Check sheet for the modelled part. Datum: model origin and axes. Units: mm. Face numbers are marked on the shaded views. A direction names the side the tool comes from. Give positions to 0.01 mm unless a question says otherwise; leave off trailing zeros. Loops run counter-clockwise (first coordinate to the right, second up) from the corner with the lowest first, then second, coordinate; pieces in that order, holes last. Notation, with made-up numbers: M 73.5,89.5 L 87.5,89.5 A27 cw 87.5,128.5 Z; hole C 74.25,-22.5 d11. An arc over 180 degrees is marked long. Write each question's results on one line, items separated by ' | '. Start each with the question number.
1. Sectioned sample at C-C on y = 54. Record the cut outline in (x, z), and give its area (3 significant figures).
2. Draft check along Z on the marked faces 3 and 4. Enter one of: pulls with the +Z half, pulls with the -Z half, needs draft (parallel to the pull), parting line crosses it, or undercut.
3. Tool access check on the marked faces 1 and 2. Record the directions out of +Z, -Z, +X, -X, +Y, -Y that give a thin tool (end or side, any length) a straight path to the whole face; none if there is none.
4. Sectioned sample at B-B on z = 20. Record the cut outline in (x, y), and give its area (3 significant figures).
5. Sectioned sample at D-D on x = -20. Record the cut outline in (y, z), and give its area (3 significant figures).
6. Sectioned sample at A-A on x = 0. Give the number of separate pieces and of enclosed holes in the cut face, and give its area (3 significant figures).
7. Material ranges on line 1 along X through (y, z) = (124.9, 0); line 2 along X through (y, z) = (39.5, 0); line 3 along Y through (x, z) = (22, 1), recorded low to high.
8. Go/stop test with flat-tipped pins: pin 1 (10 mm diameter, centred on x = 12, y = 100, fed in from -Z); pin 2 (15.5 mm diameter, centred on x = 0, z = 0, fed in from -Y); pin 3 (3 mm diameter, centred on x = -9.5, y = 84, fed in from +Z). Record where each tip stops, or that it passes through.
```python
from build123d import *

# Parameters (mm, degrees)
SKETCH2_R           = 37.5
BOSS_EXTRUDE1_DEPTH = 2
SKETCH4_R           = 15
BOSS_EXTRUDE2_DEPTH = 61
SKETCH5_R           = 25
BOSS_EXTRUDE3_DEPTH = 3
CUT_EXTRUDE1_REACH  = 139.628
SKETCH6_R           = 1.5
CUT_EXTRUDE2_REACH  = 139.628
SKETCH7_R           = 1.5
SHELL1_OUTLINE_R    = 13
SHELL1_DEPTH        = 125


# Read off the part's stored shape, not the designer's step: Shell1
with BuildPart() as part:
    # Sketch2 → Boss-Extrude1 (new body)
    with BuildSketch(Plane(origin=(0, 0, 0), x_dir=(1, 0, 0), z_dir=(0, 1, 0))):
        with Locations(Location((0, 0, 0), (0, 0, 270))):
            Circle(SKETCH2_R)
    extrude(amount=BOSS_EXTRUDE1_DEPTH)

    # Sketch4 → Boss-Extrude2 (add)
    with BuildSketch(Plane(origin=(0, 2, 0), x_dir=(1, 0, 0), z_dir=(0, 1, 0))):
        with Locations(Location((0, 0, 0), (0, 0, 90))):
            Circle(SKETCH4_R)
    boss_extrude2 = extrude(amount=BOSS_EXTRUDE2_DEPTH)

    # Mirror1: Boss-Extrude2 across plane
    add(boss_extrude2.mirror(Plane.ZX.offset(63)))

    # Sketch5 → Boss-Extrude3 (add)
    with BuildSketch(Plane(origin=(0, 124, 0), x_dir=(1, 0, 0), z_dir=(0, 1, 0))):
        with Locations(Location((0, 0, 0), (0, 0, 270))):
            Circle(SKETCH5_R)
    extrude(amount=BOSS_EXTRUDE3_DEPTH)

    # Sketch6 → Cut-Extrude1 (cut, up to next)
    with BuildSketch(Plane(origin=(0, 127, 0), x_dir=(1, 0, 0), z_dir=(0, 1, 0)), mode=Mode.PRIVATE) as cut_extrude1_sk1:
        with Locations(Location((0, 20, 0), (0, 0, 270))):
            Circle(SKETCH6_R)
    cut_extrude1_tool1 = extrude(cut_extrude1_sk1.sketch, amount=-CUT_EXTRUDE1_REACH, mode=Mode.PRIVATE) & part.part
    # Sketch6 → Cut-Extrude1 (cut, up to next)
    with BuildSketch(Plane(origin=(0, 127, 0), x_dir=(1, 0, 0), z_dir=(0, 1, 0)), mode=Mode.PRIVATE) as cut_extrude1_sk2:
        with Locations(Location((20, 0, 0), (0, 0, 270))):
            Circle(SKETCH6_R)
    cut_extrude1_tool2 = extrude(cut_extrude1_sk2.sketch, amount=-CUT_EXTRUDE1_REACH, mode=Mode.PRIVATE) & part.part
    # Sketch6 → Cut-Extrude1 (cut, up to next)
    with BuildSketch(Plane(origin=(0, 127, 0), x_dir=(1, 0, 0), z_dir=(0, 1, 0)), mode=Mode.PRIVATE) as cut_extrude1_sk3:
        with Locations(Location((0, -20, 0), (0, 0, 270))):
            Circle(SKETCH6_R)
    cut_extrude1_tool3 = extrude(cut_extrude1_sk3.sketch, amount=-CUT_EXTRUDE1_REACH, mode=Mode.PRIVATE) & part.part
    # Sketch6 → Cut-Extrude1 (cut, up to next)
    with BuildSketch(Plane(origin=(0, 127, 0), x_dir=(1, 0, 0), z_dir=(0, 1, 0)), mode=Mode.PRIVATE) as cut_extrude1_sk4:
        with Locations(Location((-20, 0, 0), (0, 0, 270))):
            Circle(SKETCH6_R)
    cut_extrude1_tool4 = extrude(cut_extrude1_sk4.sketch, amount=-CUT_EXTRUDE1_REACH, mode=Mode.PRIVATE) & part.part
    add(cut_extrude1_tool1.solids().sort_by_distance((0, 127, -20))[0], mode=Mode.SUBTRACT)
    add(cut_extrude1_tool2.solids().sort_by_distance((20, 127, 0))[0], mode=Mode.SUBTRACT)
    add(cut_extrude1_tool3.solids().sort_by_distance((0, 127, 20))[0], mode=Mode.SUBTRACT)
    add(cut_extrude1_tool4.solids().sort_by_distance((-20, 127, 0))[0], mode=Mode.SUBTRACT)

    # Sketch7 → Cut-Extrude2 (cut, up to next)
    with BuildSketch(Plane.XZ, mode=Mode.PRIVATE) as cut_extrude2_sk1:
        with Locations(Location((0, 32.5, 0), (0, 0, 270))):
            Circle(SKETCH7_R)
    cut_extrude2_tool1 = extrude(cut_extrude2_sk1.sketch, amount=-CUT_EXTRUDE2_REACH, mode=Mode.PRIVATE) & part.part
    # Sketch7 → Cut-Extrude2 (cut, up to next)
    with BuildSketch(Plane.XZ, mode=Mode.PRIVATE) as cut_extrude2_sk2:
        with Locations(Location((32.5, 0, 0), (0, 0, 270))):
            Circle(SKETCH7_R)
    cut_extrude2_tool2 = extrude(cut_extrude2_sk2.sketch, amount=-CUT_EXTRUDE2_REACH, mode=Mode.PRIVATE) & part.part
    # Sketch7 → Cut-Extrude2 (cut, up to next)
    with BuildSketch(Plane.XZ, mode=Mode.PRIVATE) as cut_extrude2_sk3:
        with Locations(Location((0, -32.5, 0), (0, 0, 270))):
            Circle(SKETCH7_R)
    cut_extrude2_tool3 = extrude(cut_extrude2_sk3.sketch, amount=-CUT_EXTRUDE2_REACH, mode=Mode.PRIVATE) & part.part
    # Sketch7 → Cut-Extrude2 (cut, up to next)
    with BuildSketch(Plane.XZ, mode=Mode.PRIVATE) as cut_extrude2_sk4:
        with Locations(Location((-32.5, 0, 0), (0, 0, 270))):
            Circle(SKETCH7_R)
    cut_extrude2_tool4 = extrude(cut_extrude2_sk4.sketch, amount=-CUT_EXTRUDE2_REACH, mode=Mode.PRIVATE) & part.part
    add(cut_extrude2_tool1.solids().sort_by_distance((0, 0, 32.5))[0], mode=Mode.SUBTRACT)
    add(cut_extrude2_tool2.solids().sort_by_distance((32.5, 0, 0))[0], mode=Mode.SUBTRACT)
    add(cut_extrude2_tool3.solids().sort_by_distance((0, 0, -32.5))[0], mode=Mode.SUBTRACT)
    add(cut_extrude2_tool4.solids().sort_by_distance((-32.5, 0, 0))[0], mode=Mode.SUBTRACT)

    # Shell1 outline → Shell1 (cut)
    with BuildSketch(Plane(origin=(0, 0, 0), x_dir=(1, 0, 0), z_dir=(0, 1, 0))):
        Circle(SHELL1_OUTLINE_R)
    extrude(amount=SHELL1_DEPTH, mode=Mode.SUBTRACT)


solid = part.part
```
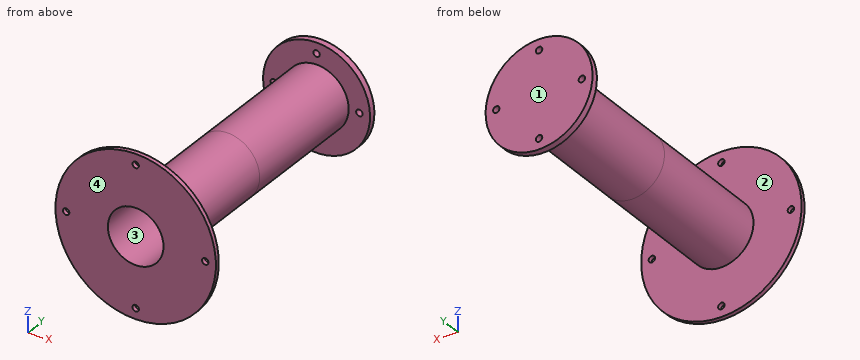
Output values:
1) outline: C 0,0 d30; hole C 0,0 d26 | area: 176 mm2
2) face 3: undercut | face 4: needs draft
3) face 1: +Z, -Z, +X, -X, +Y | face 2: none
4) outline: M -31.72,0 L 31.72,0 L 31.72,2 L -31.72,2 Z; M -15,124 L -1.5,124 L -1.5,127 L -15,127 Z; M 1.5,124 L 15,124 L 15,127 L 1.5,127 Z | area: 208 mm2
5) outline: M 0,-31.72 L 2,-31.72 L 2,31.72 L 0,31.72 Z; M 124,-15 L 127,-15 L 127,-1.5 L 124,-1.5 Z; M 124,1.5 L 127,1.5 L 127,15 L 124,15 Z | area: 208 mm2
6) separate pieces: 5 | enclosed holes: 0 | area: 680 mm2
7) line 1: -25 to -21.5, -18.5 to -13, 13 to 18.5, 21.5 to 25 | line 2: -15 to -13, 13 to 15 | line 3: 0 to 2, 124 to 127
8) pin 1: z = -13.27 | pin 2: y = 125 | pin 3: z = 12.69
